CAD build for the part. Positions are in the model's coordinates, mm. A direction names the side the tool comes from. Round coordinates to 2 decimals unless told otherwise and drop trailing zeros. Order: outer loops, then holes, each group sorted by start corner. A loop starts at its lowest first (then second) coordinate and runs counter-clockwise, first axis right, second up. Notation, with made-up numbers: (39.5, 44) -> (64.5, 44) arc R21 cw to (64.5, 55) -> close; hole circle Ø2 at (-19.75, -16). An arc over 180 degrees is marked (long way). Return JSON: item names as keys, results as strings. Group by question number.
Q1. Which spindle directions (+Z, -Z, +X, -X, +Y, -Y) get a long thin tool onto all of the face, cutting with end or side? Do faces 4 (the flat face through (-235.665, 9.86, -374.386)), 5 (the flat face through (-182, 10, 0)). Say none if no direction does.
Q2. Mould opens along X. For faces 1 (the flat face through (-32.006, 9.86, -69.26)), 2 (the flat face through (-54.065, 10, -245)), 3 (the cylindrical face through (18.12, 10.14, -299.73)) say: +X half, -X half, draft (parallel to the pull), parting line (faces both ways), or undercut.
Q3. Cut at C-C (y = 13.25). Count the separate pieces of the cut face and the enclosed holes in it, then the cut area to 3 significant figures.
Q4. Cut at A-A (z = -211). Write the cut outline in (x, y).
Q5. Probe line 1 along X through (y, z) = (2, -269.5); line 2 along Z through (x, y) = (-163, 13.75); line 3 along Z through (x, y) = (-162.5, 18). List the from-to ranges inside material, lowest first.
Q6. Cut at B-B (z = -466.5). Write the cut outline in (x, y).
Q7. Flat gauge pins, fed straight in: pin 1 (4 mm diameter, centred on x = -28, y = 4, fed in from +Z); pin 2 (3 mm diameter, centred on y = 4, z = -380.5, fed in from -X); pin 3 (10 mm diameter, centred on x = -230, y = 13, fed in from -Z). Where does each tip first touch, or does it go through?
from build123d import *

# Parameters (mm, degrees)
SKETCH1_R           = 40.52203667
SKETCH1_W           = 43.509433639
SKETCH1_H           = 49.835103658
SKETCH1_H_2         = 48.542170344
SKETCH1_W_2         = 43.509433638
BOSS_EXTRUDE6_DEPTH = 20
FILLET1_R           = 30
FILLET2_R           = 30


with BuildPart() as part:
    # Sketch1 → Boss-Extrude6 (new body)
    with BuildSketch(Plane(origin=(0, 0, 0), x_dir=(1, 0, 0), z_dir=(0, 1, 0))):
        Polygon((-324.500042801, 0), (-36.61106831, 0), (-36.61106831, -72.630227613), (19.444444444, -30.98937664), (19.444444444, 0), (19.444444444, 300), (-180.555555556, 600), (-380.555555556, 300), (-380.555555556, 0), (-380.555555556, -30.98937664), (-324.500042801, -72.630227613), align=None)
        with Locations((-180.555555556, 199.47796333)):
            Circle(SKETCH1_R, mode=Mode.SUBTRACT)
        Polygon((-350.555555556, 98.955926659), (-307.046121917, 98.955926659), (-350.555555556, 40.384990781), align=None, mode=Mode.SUBTRACT)
        Polygon((-218.052993309, 18.381237109), (-277.907920592, 98.955926659), (-83.203190519, 98.955926659), (-143.058117802, 18.381237109), align=None, mode=Mode.SUBTRACT)
        Polygon((-40.212760909, 30), (-97.055418804, 30), (-68.634089856, 68.259836918), align=None, mode=Mode.SUBTRACT)
        with Locations((-328.800838736, 153.873478488)):
            Rectangle(SKETCH1_W, SKETCH1_H, mode=Mode.SUBTRACT)
        Polygon((-194.895952536, 524.406135398), (-246.308768225, 447.286911864), (-194.895952536, 447.286911864), align=None, mode=Mode.SUBTRACT)
        Polygon((-36.61106831, 330), (-96.633315679, 420.033371054), (-153.463987032, 330), align=None, mode=Mode.SUBTRACT)
        Polygon((-324.500042801, 330), (-207.64712408, 330), (-264.477795432, 420.033371054), align=None, mode=Mode.SUBTRACT)
        Polygon((-10.555555556, 40.384990781), (-54.064989194, 98.955926659), (-10.555555556, 98.955926659), align=None, mode=Mode.SUBTRACT)
        with Locations((-328.800838736, 245.728914828)):
            Rectangle(SKETCH1_W, SKETCH1_H_2, mode=Mode.SUBTRACT)
        with Locations((-32.310272375, 153.873478488)):
            Rectangle(SKETCH1_W_2, SKETCH1_H, mode=Mode.SUBTRACT)
        Polygon((-320.898350202, 30), (-264.055692307, 30), (-292.477021255, 68.259836918), align=None, mode=Mode.SUBTRACT)
        with Locations((-32.310272375, 245.728914828)):
            Rectangle(SKETCH1_W_2, SKETCH1_H_2, mode=Mode.SUBTRACT)
        with BuildLine():
            Line((-279.511482215, 270), (-279.511482215, 221.457829656))
            Line((-279.511482215, 221.457829656), (-247.564832021, 221.457829656))
            ThreePointArc((-247.564832021, 221.457829656), (-232.312774166, 247.379403578), (-207.64712408, 264.58867344))
            Line((-207.64712408, 264.58867344), (-207.64712408, 270))
            Line((-207.64712408, 270), (-279.511482215, 270))
        make_face(mode=Mode.SUBTRACT)
        with BuildLine():
            Line((-279.511482215, 128.955926659), (-279.511482215, 178.791030317))
            Line((-279.511482215, 178.791030317), (-247.975200012, 178.791030317))
            ThreePointArc((-247.975200012, 178.791030317), (-232.771073725, 152.076514844), (-207.64712408, 134.367253219))
            Line((-207.64712408, 134.367253219), (-207.64712408, 128.955926659))
            Line((-207.64712408, 128.955926659), (-279.511482215, 128.955926659))
        make_face(mode=Mode.SUBTRACT)
        with BuildLine():
            Line((-153.463987032, 134.367253219), (-153.463987032, 128.955926659))
            Line((-153.463987032, 128.955926659), (-81.599628896, 128.955926659))
            Line((-81.599628896, 128.955926659), (-81.599628896, 178.791030317))
            Line((-81.599628896, 178.791030317), (-113.135911099, 178.791030317))
            ThreePointArc((-113.135911099, 178.791030317), (-128.340037386, 152.076514844), (-153.463987032, 134.367253219))
        make_face(mode=Mode.SUBTRACT)
        with BuildLine():
            Line((-153.463987032, 264.58867344), (-153.463987032, 270))
            Line((-153.463987032, 270), (-81.599628896, 270))
            Line((-81.599628896, 270), (-81.599628896, 221.457829656))
            Line((-81.599628896, 221.457829656), (-113.54627909, 221.457829656))
            ThreePointArc((-113.54627909, 221.457829656), (-128.798336945, 247.379403578), (-153.463987032, 264.58867344))
        make_face(mode=Mode.SUBTRACT)
        Polygon((-114.802342886, 429.992241235), (-166.215158575, 429.992241235), (-166.215158575, 348.542048906), align=None, mode=Mode.SUBTRACT)
        Polygon((-114.802342886, 447.286911864), (-166.215158575, 524.406135398), (-166.215158575, 447.286911864), align=None, mode=Mode.SUBTRACT)
        Polygon((-246.308768225, 429.992241235), (-194.895952536, 348.542048906), (-194.895952536, 429.992241235), align=None, mode=Mode.SUBTRACT)
    extrude(amount=BOSS_EXTRUDE6_DEPTH)

    # Fillet1
    fillet1_edges = [part.edges().sort_by_distance(p)[0] for p in [
        (-180.555555556, 10, -600),
    ]]
    fillet(fillet1_edges, radius=FILLET1_R)

    # Fillet2
    fillet2_edges = [part.edges().sort_by_distance(p)[0] for p in [
        (19.444444444, 10, 30.98937664),
        (-36.61106831, 10, 0),
        (-324.500042801, 10, 0),
        (-380.555555556, 10, 30.98937664),
        (-380.555555556, 10, -300),
        (19.444444444, 10, -300),
    ]]
    fillet(fillet2_edges, radius=FILLET2_R)


solid = part.part
Solution:
{
 "1": {"face 4": "+Y, -Y", "face 5": "+Z, +Y, -Y"},
 "2": {"face 1": "undercut", "face 2": "undercut", "face 3": "+X half"},
 "3": {"separate pieces": "1", "enclosed holes": "20", "area": "128,000 mm²"},
 "4": {"outline": "(-380.56, 0) -> (-219.4, 0) -> (-219.4, 20) -> (-380.56, 20) -> close; (-141.71, 0) -> (19.44, 0) -> (19.44, 20) -> (-141.71, 20) -> close"},
 "5": {"line 1": "x = -380.56 to -350.56, -307.05 to -279.51, -207.65 to -153.46, -81.6 to -54.06, -10.56 to 19.44", "line 2": "z = -570.24 to -519.58, -447.29 to -429.99, -353.64 to -236, -162.96 to -98.96, -18.38 to 0", "line 3": "z = -569.87 to -518.83, -447.29 to -429.99, -354.43 to -235.76, -163.2 to -98.96, -18.38 to 0"},
 "6": {"outline": "(-269.56, 0) -> (-233.5, 0) -> (-233.5, 20) -> (-269.56, 20) -> close; (-194.9, 0) -> (-166.22, 0) -> (-166.22, 20) -> (-194.9, 20) -> close; (-127.61, 0) -> (-91.56, 0) -> (-91.56, 20) -> (-127.61, 20) -> close"},
 "7": {"pin 1": "stops at z = 67.72", "pin 2": "stops at x = -327.89", "pin 3": "stops at z = -533.33"}
}
